```python
from build123d import *

# Parameters (mm, degrees)
SKETCH_1_R             = 4.35
SKETCH_1_R_2           = 29.732137495
SM_BASE_FLANGE_1_DEPTH = 5
OTHER_START            = -2.7
OTHER_1_OUTLINE_W      = 20.4
OTHER_1_OUTLINE_H      = 5
OTHER_1_DEPTH          = 5.4


# Read off the part's stored shape, not the designer's step: Выступы и прорези-Прорезь1
# Sheet-metal steps are written as plain solids
with BuildPart() as part:
    # Sketch 1 → Базовая кромка1 (new body)
    with BuildSketch(Plane.XY):
        with BuildLine():
            Line((153.076706029, -3), (153.076706029, -27))
            Line((153.076706029, -27), (-47, -27))
            Line((-47, -27), (-47, -3))
            ThreePointArc((-47, -3), (-47.878679656, -0.878679656), (-50, 0))
            Line((-50, 0), (-74, 0))
            Line((-74, 0), (-74, 40))
            Line((-74, 40), (-61.150039911, 107.459829597))
            ThreePointArc((-61.150039911, 107.459829597), (-20.166822902, 154.704084341), (41.173899677, 142.499190395))
            Line((41.173899677, 142.499190395), (180.076706029, 20))
            Line((180.076706029, 20), (180.076706029, 0))
            Line((180.076706029, 0), (156.076706029, 0))
            ThreePointArc((156.076706029, 0), (153.955385686, -0.878679656), (153.076706029, -3))
        make_face()
        with Locations((-37.675, 95.811778053)):
            Circle(SKETCH_1_R, mode=Mode.SUBTRACT)
        with Locations((37.675, 95.811778053)):
            Circle(SKETCH_1_R, mode=Mode.SUBTRACT)
        with Locations((0, 95.811778053)):
            Circle(SKETCH_1_R_2, mode=Mode.SUBTRACT)
    extrude(amount=-SM_BASE_FLANGE_1_DEPTH)

    # Other 1 outline → Other 1 (cut)
    with BuildSketch(Plane.YZ.offset(OTHER_START)):
        with Locations((41.079640558, -2.5)):
            Rectangle(OTHER_1_OUTLINE_W, OTHER_1_OUTLINE_H)
        with Locations((-12, -2.5)):
            Rectangle(OTHER_1_OUTLINE_W, OTHER_1_OUTLINE_H)
    extrude(amount=OTHER_1_DEPTH, mode=Mode.SUBTRACT)


solid = part.part
```
The model under review builds one solid part; all positions refer to its coordinate system, in mm. A direction names the side the tool comes from. Round coordinates to 2 decimals unless told otherwise and drop trailing zeros. Write each loop counter-clockwise with the first axis right and the second up, starting at its lowest first coordinate (ties: lowest second). Pieces come first, ordered by that corner, then holes. Notation, with made-up numbers: M 77.25,68.25 L 107.25,68.25 A23 cw 107.25,85.25 Z; hole C -26,-14.75 d3. An arc over 180 degrees is marked long. Use CSV: the item, a comma, the result in double quotes. Start each with the question number.
(1) Clearance check with flat-ended pins moving along their axes: P1, Ø2.5, axis at y = -15.5, z = -2.5, coming from the +X side; P2, Ø2.5, axis at y = -9.5, z = -3, coming from the -X side; P3, Ø1.5, axis at x = -64, z = -3.5, coming from the -Y side. State where each tip first meets the part, or that it passes through.
(2) We need section C-C, the plane z = -3.35. State the section outline as (x, y) points (3 decimals).
(3) The part is to be moulded in two halves that separate along Y. For faces 1 (the face through (109.65, 82.11, -2.46)), 2 (the face through (27, 46, 0)), 3 (the face through (39.68, 91.95, -2.46)), say which applies: +Y half, -Y half, draft (parallel to the pull), parting line (faces both ways), or undercut.
(4) Tool access review of faces 4 (the face through (153.077, -15, -2)), 5 (the face through (-21.03, 154.4, -2.46)), 6 (the face through (-62, 0, -2)), 7 (the face through (-74, 20, -2)), 8 (the face through (0, 51.28, -3)): name each direction out of +Z, -Z, +X, -X, +Y, -Y from which nothing blocks a thin tool from reaching the whole face with its end or side.
(5) We need section A-A, the plane x = 0. State the section outline as (y, z) points, then the cut area to 3 significant figures.
(6) We need section D-D, the plane y = 75. State the section outline as (x, z) points.
(7) For line 1 along Y through (x, z) = (0.5, -1.3); line 2 along X through (y, z) = (-9.5, -0.9); line 3 along X through (y, z) = (39, -3.9), list the stretches that pass through material, from the lowest coordinate up.
(8) We need section B-B, the plane y = -8. State the section outline as (x, z) points, then the cut area to 3 significant figures.
Findings:
1,P1,"x = 153.08"
1,P2,"x = -47"
1,P3,"y = 0"
2,outline,"M -74,0 L -50,0 A3 cw -47,-3 L -47,-27 L 153.077,-27 L 153.077,-3 A3 cw 156.077,0 L 180.077,0 L 180.077,20 L 41.174,142.499 A62.25 ccw -61.15,107.46 L -74,40 Z; hole C -37.675,95.812 d8.7; hole C 0,95.812 d59.464; hole M -2.7,-22.2 L 2.7,-22.2 L 2.7,-1.8 L -2.7,-1.8 Z; hole M -2.7,30.88 L 2.7,30.88 L 2.7,51.28 L -2.7,51.28 Z; hole C 37.675,95.812 d8.7"
3,face 1,"+Y half"
3,face 2,"draft"
3,face 3,"undercut"
4,face 4,"+Z, -Z, +X, -Y"
4,face 5,"+Z, -Z, +Y"
4,face 6,"+Z, -Z, -X, -Y"
4,face 7,"+Z, -Z, -X, +Y, -Y"
4,face 8,"+Z, -Z"
5,outline,"M -27,-5 L -22.2,-5 L -22.2,0 L -27,0 Z; M -1.8,-5 L 30.88,-5 L 30.88,0 L -1.8,0 Z; M 51.28,-5 L 66.08,-5 L 66.08,0 L 51.28,0 Z; M 125.54,-5 L 158.06,-5 L 158.06,0 L 125.54,0 Z"
5,area,"424 mm^2"
6,outline,"M -67.33,-5 L -21.23,-5 L -21.23,0 L -67.33,0 Z; M 21.23,-5 L 117.71,-5 L 117.71,0 L 21.23,0 Z"
7,line 1,"-27 to -22.2, -1.8 to 30.88, 51.28 to 66.08, 125.54 to 158.06"
7,line 2,"-47 to -2.7, 2.7 to 153.08"
7,line 3,"-74 to -2.7, 2.7 to 158.53"
8,outline,"M -47,-5 L -2.7,-5 L -2.7,0 L -47,0 Z; M 2.7,-5 L 153.08,-5 L 153.08,0 L 2.7,0 Z"
8,area,"973 mm^2"
